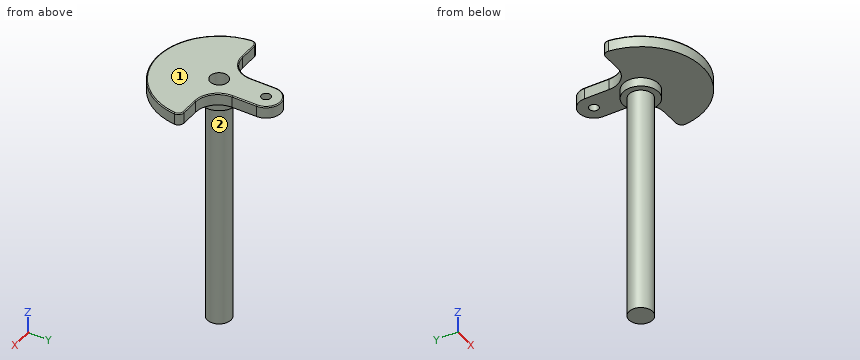
Autodesk Inventor part; units mm, degrees
ref_plane "YZ Plane" through (0, 0, 0) normal (1, 0, 0) x (0, 1, 0)
ref_plane "XZ Plane" through (0, 0, 0) normal (0, 1, 0) x (-1, 0, 0)
ref_plane "XY Plane" through (0, 0, 0) normal (0, 0, 1) x (1, 0, 0)
sketch "Boceto1" plane through (0, 0, 0) normal (0, 0, 1) x (1, 0, 0)
  circle A0 centre (0, 0) radius 2.3813
  arc A1 (4.0409, 12.7) -> (-4.0409, 12.7) centre (0, 12.7) ccw
  arc A2 (-10.1023, 0) -> (-4.0409, 6.0614) centre (-10.1023, 6.0614) ccw
  line L0 (-4.0409, 12.7) -> (-4.0409, 6.0614)
  line L1 (4.0409, 12.7) -> (4.0409, 6.0614)
  arc A3 (4.0409, 6.0614) -> (10.1023, 0) centre (10.1023, 6.0614) ccw
  arc A4 (-15.0775, 0) -> (-16.5852, -1.6669) centre (-15.0775, -1.5153) ccw
  line L2 (-23.7372, 0) -> (23.7372, 0) construction
  arc A5 (16.5852, -1.6669) -> (15.0775, 0) centre (15.0775, -1.5153) ccw
  arc A6 (-16.5852, -1.6669) -> (16.5852, -1.6669) centre (0, 0) ccw
  line L3 (10.1023, 0) -> (15.0775, 0)
  line L4 (-15.0775, 0) -> (-10.1023, 0)
  dimension "d1" = 4.7625
  dimension "d2" = 8.0818
  dimension "d3" = 12.1227
  dimension "d5" = 12.7
  dimension "d6" = 3.0307
extrude "Extrusión1" add sketch "Boceto1" against normal blind 3.175
sketch "Boceto2" plane through (0, 0, 0) normal (0, 0, 1) x (1, 0, 0)
  line L0 (0, 0) -> (0, 12.7) construction
  line L1 (0, 0) -> (12.7, 0) construction
  dimension "d9" = 12.7
  dimension "d10" = 90
hole "Agujero1" at (0, 12.7, 0) direction (0, 0, -1) diameter 2.4867 end through all
sketch "Boceto3" plane through (0, 0, -3.175) normal (0, 0, -1) x (-1, 0, 0)
  circle A0 centre (0, 0) radius 4.7625
  circle A1 centre (0, 0) radius 2.3813
  dimension "d18" = 9.525
  dimension "d19" = 4.7625
extrude "Extrusión2" add sketch "Boceto3" along normal blind 2.3813
sketch "Boceto4" plane through (0, 0, -5.5563) normal (0, 0, -1) x (-1, 0, 0)
  circle A0 centre (0, 0) radius 3.175
  dimension "d22" = 6.35
extrude "Extrusión3" add sketch "Boceto4" along normal blind 61.9125
fillet "Empalme1" radius 0.254 10 edges at (-4.0409, 9.3807, 0) (-5.8162, 1.7753, 0) (-12.5899, 0, 0) (-16.2013, -0.4988, 0) (0, -16.6688, 0) (16.2013, -0.4988, 0) (12.5899, 0, 0) (5.8162, 1.7753, 0) (4.0409, 9.3807, 0) (0, 16.7409, 0)
properties part number "CrankShaft"
Geometry check sheet. Reference: the model listing, model coordinates, mm. Face numbers are marked on the shaded views. A direction names the side the tool comes from. Round coordinates to 2 decimals unless told otherwise and drop trailing zeros. Loops run counter-clockwise (first coordinate to the right, second up) from the corner with the lowest first, then second, coordinate; pieces in that order, holes last. Notation, with made-up numbers: (22, -35) - (41, -35) arc R10 ccw to (41, -31) - close; hole circle Ø8 at (24, 60). An arc over 180 degrees is marked (long way). One line per question, with ' | ' between items. Start each with the question number.
1. Tool access check on the marked faces 1 and 2. Record the directions out of +Z, -Z, +X, -X, +Y, -Y that give a thin tool (end or side, any length) a straight path to the whole face; none if there is none.
2. Depth check by flat-ended pin: pin 1 (1.5 mm diameter, centred on y = -0.5, z = -12, fed in from -X) (3 decimals); pin 2 (12 mm diameter, centred on x = -2, z = -23.5, fed in from +Y) (3 decimals); pin 3 (6 mm diameter, centred on x = 0, y = 0, fed in from +Z); pin 4 (1.5 mm diameter, centred on x = -13.5, z = -1.5, fed in from +Y). Enter the tip coordinate at first touch or a pass-through.
3. Scan lines: line 1 (Y direction, x = 0, z = -1); line 2 (X direction, y = 12.7, z = -2.25); line 3 (Z direction, x = 5.5, y = -2.5) (3 decimals). Record each from-to range of solid material in increasing order. Write a range as [from, to].
4. Cross-section at C-C on z = -43.5. Record the cut outline in (x, y) (3 decimals).
5. Cross-section at B-B on y = 7. Record the cut outline in (x, z) (3 decimals), then the cut area to 3 significant figures.
Taken from the geometry:
1) face 1: +Z, +X, -X, +Y, -Y | face 2: -Z
2) pin 1: x = -3.175 | pin 2: y = 3.175 | pin 3: z = 0 | pin 4: y = 0
3) line 1: [-16.67, -2.38], [2.38, 11.46], [13.94, 16.74] | line 2: [-4.04, -1.24], [1.24, 4.04] | line 3: [-3.175, 0]
4) outline: circle Ø6.35 at (0, 0)
5) outline: (-4.041, -3.175) - (4.041, -3.175) - (4.041, -0.254) arc R0.254 ccw to (3.787, 0) - (-3.787, 0) arc R0.254 ccw to (-4.041, -0.254) - close | area: 25.6 mm²
